Input: dimensioned drawing with shaded views. Units: mm. Origin: part minimum x, y, z. A direction names the side the tool comes from. Round coordinates to 2 decimals unless told otherwise and drop trailing zeros. Order: outer loops, then holes, each group sorted by start corner. A loop starts at its lowest first (then second) coordinate and runs counter-clockwise, first axis right, second up. Notation, with made-up numbers: M 61,85.25 L 118,85.25 A11 ccw 118,91.25 Z; hole C 88,-33.75 d6. An arc over 180 degrees is marked long. Put each result on its own line as item: value. Start each with the question number.
1) Access query for the marked faces 1, 2, 3, 4 and 5. Directions: +Z, -Z, +X, -X, +Y, -Y. A direction counts if a zero-diameter tool reaches every point of the face in a straight line with its end or side. Return the directions, or none.
2) Section D-D, the plane x = 2.5. Return loops of the section in (y, z), then the cut area to 3 significant figures.
3) Material intervals for probe 1 along Y at (x, z) = (22, 3.5); probe 2 along Z at (x, y) = (8.25, 6.5); probe 3 along X at (y, z) = (6.75, 7.25) (1 decimal), sorted ascending. Write a range as [from, to].
4) Section A-A, the plane y = 9. Return loops of the section in (x, z).
5) Section B-B, the plane z = 4. Return loops of the section in (x, y), then the cut area to 3 significant figures.
6) Section C-C, the plane x = 23.75. Return loops of the section in (y, z), then the cut area to 3 significant figures.
7) First-contact query: P1, Ø1, axis at x = 12, y = 7, coming from the -Z side; P2, Ø5, axis at x = 7.5, y = 6.5, coming from the +Z side; P3, Ø2, axis at y = 8.5, z = 6.5, coming from the +X side. Flat tips, straight axial feed; report the tip coordinate or a pass-through.
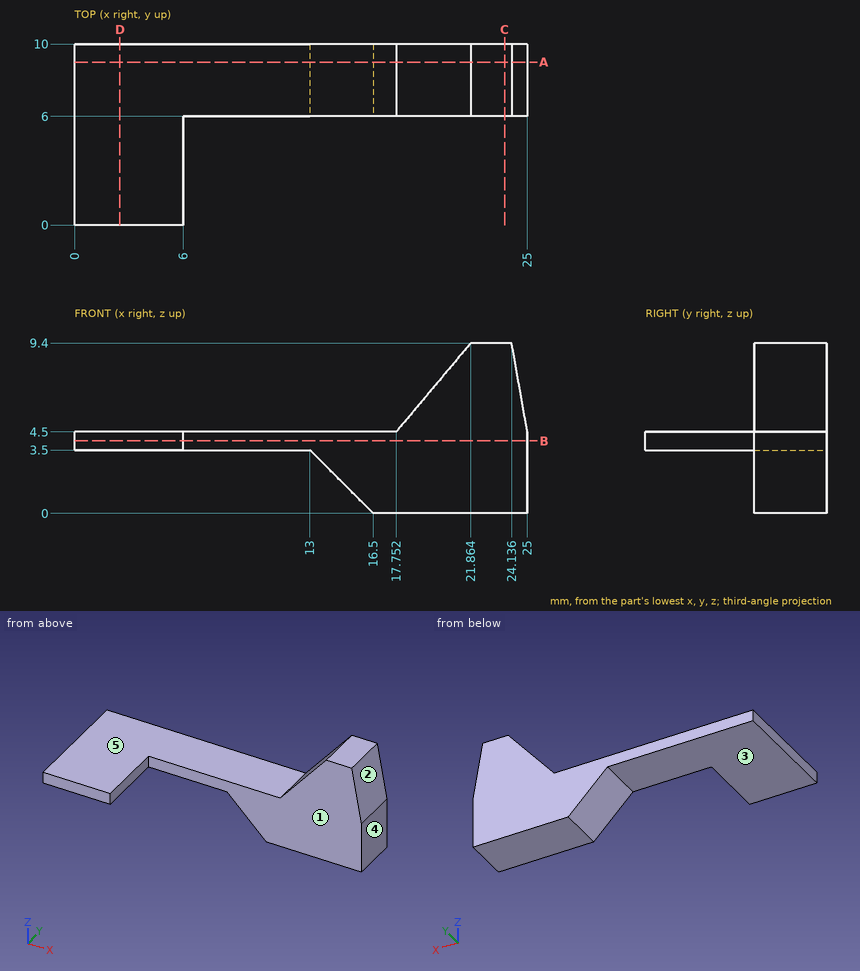
Result sheet:
1. face 1: +Z, -Z, +X, -Y
1. face 2: +Z, +X, +Y, -Y
1. face 3: -Z, -X, +Y, -Y
1. face 4: +Z, -Z, +X, +Y, -Y
1. face 5: +Z, -X, +Y, -Y
2. outline: M 0,3.5 L 10,3.5 L 10,4.5 L 0,4.5 Z
2. area: 10.0 mm2
3. probe 1: y = [6, 10]
3. probe 2: z = [3.5, 4.5]
3. probe 3: x = [20.1, 24.5]
4. outline: M 0,3.5 L 13,3.5 L 16.5,0 L 25,0 L 25,4.5 L 24.14,9.4 L 21.86,9.4 L 17.75,4.5 L 0,4.5 Z
5. outline: M 0,0 L 6,0 L 6,6 L 25,6 L 25,10 L 0,10 Z
5. area: 136 mm2
6. outline: M 6,0 L 10,0 L 10,9.4 L 6,9.4 Z
6. area: 37.6 mm2
7. P1: stops at z = 3.5
7. P2: stops at z = 4.5
7. P3: stops at x = 24.82
